The listing builds one solid part. Answer for the finished solid, in the listing's coordinates (mm). Face numbers are marked on the shaded views. A direction names the side the tool comes from. Give positions to 0.01 mm unless a question says otherwise; leave off trailing zeros. Order: outer loops, then holes, each group sorted by start corner. A loop starts at its lowest first (then second) coordinate and runs counter-clockwise, first axis right, second up. Notation, with made-up numbers: (-2, -34.5) - (41, -34.5) arc R28 ccw to (41, -16.5) - close; hole circle Ø8 at (51.5, 78). An arc over 180 degrees is marked (long way). Answer in a Markdown table with one row per item.
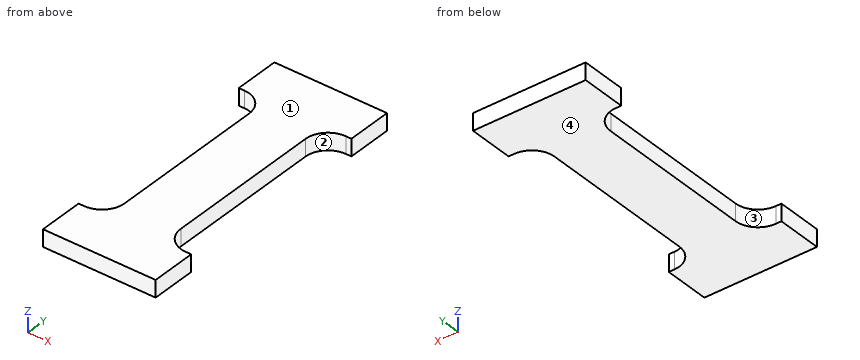
from build123d import *

# Parameters (mm, degrees)
F1_DEPTH = 1.5


with BuildPart() as f1:
    # F0 (on Top) → F1 (new body)
    with BuildSketch(Plane.XY):
        with BuildLine():
            Line((-2.5, 0), (0, 0))
            Line((0, 0), (0, 13))
            Line((0, 13), (-5, 13))
            Line((-5, 13), (-5, 9))
            Line((-5, 9), (-4.5, 9))
            ThreePointArc((-4.5, 9), (-3.085786, 8.414214), (-2.5, 7))
            Line((-2.5, 7), (-2.5, 0))
        make_face()
        with BuildLine():
            Line((0, 13), (0, 0))
            Line((0, 0), (2.5, 0))
            Line((2.5, 0), (2.5, 7))
            ThreePointArc((2.5, 7), (3.085786, 8.414214), (4.5, 9))
            Line((4.5, 9), (5, 9))
            Line((5, 9), (5, 13))
            Line((5, 13), (0, 13))
        make_face()
        with BuildLine():
            Line((0, -13), (0, 0))
            Line((0, 0), (-2.5, 0))
            Line((-2.5, 0), (-2.5, -7))
            ThreePointArc((-2.5, -7), (-3.085786, -8.414214), (-4.5, -9))
            Line((-4.5, -9), (-5, -9))
            Line((-5, -9), (-5, -13))
            Line((-5, -13), (0, -13))
        make_face()
        with BuildLine():
            Line((2.5, 0), (0, 0))
            Line((0, 0), (0, -13))
            Line((0, -13), (5, -13))
            Line((5, -13), (5, -9))
            Line((5, -9), (4.5, -9))
            ThreePointArc((4.5, -9), (3.085786, -8.414214), (2.5, -7))
            Line((2.5, -7), (2.5, 0))
        make_face()
    extrude(amount=F1_DEPTH)


solid = f1.part
Item 1: Find section C-C on y = -2.5. Write down the section's boundary in (x, z).
Answer block:
| item | result |
|---|---|
| outline | (-2.5, 0) - (2.5, 0) - (2.5, 1.5) - (-2.5, 1.5) - close |
Item 2: Which of the six approach directions +Z, -Z, +X, -X, +Y, -Y give full straight-line access (tool end or side, diameter ignored) to the marked faces 3 and 4?
Answer block:
| item | result |
|---|---|
| face 3 | +Z, -Z, -X |
| face 4 | -Z, +X, -X, +Y, -Y |
Item 3: Determine the mould class of the marked faces 1 and 2 for opening direction Y: pulls with the +Y half, pulls with the -Y half, needs draft (parallel to the pull), parting line crosses it, or undercut.
Answer block:
| item | result |
|---|---|
| face 1 | needs draft |
| face 2 | undercut |
Item 4: Find section D-D on x = 4.25. Write down the section's boundary in (y, z), then the cut area to 3 significant figures.
Answer block:
| item | result |
|---|---|
| outline | (-13, 0) - (-8.98, 0) - (-8.98, 1.5) - (-13, 1.5) - close; (8.98, 0) - (13, 0) - (13, 1.5) - (8.98, 1.5) - close |
| area | 12.0 mm² |
Item 5: Find section B-B on z = 1.05. Write down the section's boundary in (x, y), then the cut area to 3 significant figures.
Answer block:
| item | result |
|---|---|
| outline | (-5, -13) - (5, -13) - (5, -9) - (4.5, -9) arc R2 cw to (2.5, -7) - (2.5, 7) arc R2 cw to (4.5, 9) - (5, 9) - (5, 13) - (-5, 13) - (-5, 9) - (-4.5, 9) arc R2 cw to (-2.5, 7) - (-2.5, -7) arc R2 cw to (-4.5, -9) - (-5, -9) - close |
| area | 173 mm² |
Item 6: Consider line 1 (Y direction, x = -4.5, z = 0.55); line 2 (Y direction, x = -2.75, z = 0.8); line 3 (X direction, y = 5.5, z = 0.5). Determine where each line is inside the solid, lowest interval first.
Answer block:
| item | result |
|---|---|
| line 1 | -13 to -9, 9 to 13 |
| line 2 | -13 to -7.97, 7.97 to 13 |
| line 3 | -2.5 to 2.5 |
Item 7: Each of these flat-tipped pins is pushed along its axis until it touches: P1, Ø0.8, axis at y = -2, z = 1, coming from the -X side; P2, Ø0.8, axis at y = 0, z = 1, coming from the +X side. Where does it stop, or does it pass through?
Answer block:
| item | result |
|---|---|
| P1 | x = -2.5 |
| P2 | x = 2.5 |
Item 8: Find section A-A on x = -4. Write down the section's boundary in (y, z), then the cut area to 3 significant figures.
Answer block:
| item | result |
|---|---|
| outline | (-13, 0) - (-8.94, 0) - (-8.94, 1.5) - (-13, 1.5) - close; (8.94, 0) - (13, 0) - (13, 1.5) - (8.94, 1.5) - close |
| area | 12.2 mm² |
